Autodesk Inventor part; units mm, degrees
ref_plane "YZ Plane" through (0, 0, 0) normal (1, 0, 0) x (0, 1, 0)
ref_plane "XZ Plane" through (0, 0, 0) normal (0, 1, 0) x (-1, 0, 0)
ref_plane "XY Plane" through (0, 0, 0) normal (0, 0, 1) x (1, 0, 0)
sketch "Sketch1" plane through (0, 0, 0) normal (0, 0, 1) x (1, 0, 0)
  arc A0 (0.1634, -91.6592) -> (286.7211, -56.9812) centre (0.1634, 1109.6463) ccw
  arc A1 (0.1634, -106.6592) -> (276.3881, -74.8786) centre (0.1634, 1109.6463) ccw
  line L0 (286.7211, -56.9812) -> (276.3881, -74.8786)
  line L1 (286.7211, -56.9812) -> (307.3872, -56.9812) construction
  line L2 (0.1634, -106.6592) -> (0.1634, -82.9582)
  arc A2 (-286.3942, -56.9812) -> (0.1634, -91.6592) centre (0.1634, 1109.6463) ccw
  arc A3 (-276.0612, -74.8786) -> (0.1634, -106.6592) centre (0.1634, 1109.6463) ccw
  line L3 (-286.3942, -56.9812) -> (-276.0612, -74.8786)
  point P0 (0, 0)
  point P1 (254.828, -79.7002)
  dimension "d0" = 15
  dimension "d1" = 120
extrude "Extrusion1" add sketch "Sketch1" along normal blind 30
fillet "Fillet1" radius 3 12 edges at (-144.1607, -82.9582, 30) (139.1869, -98.6879, 30) (144.4876, -82.9582, 0) (286.7211, -56.9812, 15) (281.5546, -65.9299, 0) (281.5546, -65.9299, 30) (276.3881, -74.8786, 15) (139.1869, -98.6879, 0) (-286.3942, -56.9812, 15) (-281.2277, -65.9299, 30) (-276.0612, -74.8786, 15) (-281.2277, -65.9299, 0)
sketch "Sketch2" plane through (0, 0, 0) normal (0, 1, 0) x (-1, 0, 0)
  line L0 (0, 0) -> (0, 15)
  circle A0 centre (0, 15) radius 5
  dimension "d5" = 15
  dimension "d6" = 10
extrude "Extrusion2" cut sketch "Sketch2" against normal blind 300
properties part number "leaf 3" material "Steel, Carbon"
CAD build for the part. Positions are in the model's coordinates, mm. A direction names the side the tool comes from. Coordinates: 2 decimals unless noted, no trailing zeros. Order: outer loops, then holes, each group sorted by start corner. A loop starts at its lowest first (then second) coordinate and runs counter-clockwise, first axis right, second up. Notation, with made-up numbers: M 80,23 L 109,23 A36 ccw 109,61 Z; hole C 27,-29 d2. An arc over 180 degrees is marked long. Write each question's results on one line, items separated by ' | '. Start each with the question number.
Q1. Cut at A-A (z = 15). List the corners of the cut face in (x, y), then the cut area to 3 significant figures.
Q2. Pull direction X, two halves, no side cores. Call faces 1 (the cylindrical face through (1.08, -99.05, 10.12)), 2 (the flat face through (-1, -95, 30)), 3 (the cylindrical face through (-279.018, -68.047, 0.902)): +X half, -X half, draft (parallel to the pull), parting line (faces both ways), or undercut.
Q3. Drill centre lines: probe 1 along Z at (x, y) = (0, -99); probe 2 along Y at (x, z) = (193, 14.5); probe 3 along Y at (x, z) = (222, 16). Where is each one in solid material? Low to high. Write a range as from..to.
Q4. Which spindle directions (+Z, -Z, +X, -X, +Y, -Y) get a long thin tool onto all of the face, cutting with end or side? Do faces 4 (the cylindrical face through (140.47, -98.54, 14.83)), 5 (the cylindrical face through (-138.724, -83.604, 14.832)). Say none if no direction does.
Q5. Flat gauge pins, fed straight in: P1, Ø2, axis at x = 149.5, y = -84, coming from the -Z side; P2, Ø1.5, axis at y = -66.5, z = 15, coming from the +X side; P3, Ø8, axis at x = 0, z = 15, coming from the +Y side. Where does each tip first touch, or does it go through?
Found:
1) outline: M -282.89,-63.05 L -276.71,-73.75 A3 ccw -274.79,-75.17 A1216.3 ccw -5,-106.65 L -5,-91.65 A1201.3 cw -279.59,-58.63 A3 ccw Z; M 5,-106.65 A1216.31 ccw 275.12,-75.17 A3 ccw 277.04,-73.75 L 283.22,-63.05 A3 ccw 279.92,-58.63 A1201.31 cw 5,-91.65 Z | area: 8,350 mm²
2) face 1: undercut | face 2: draft | face 3: -X half
3) probe 1: 0..10, 20..30 | probe 2: -91.28..-76.08 | probe 3: -86.26..-71
4) face 4: +Z, -Z, +X, -Y | face 5: +Z, -Z, +Y
5) P1: z = 0.02 | P2: x = 281.66 | P3: through
